Drawing for the job (mm, zero at the part's lowest x, y, z). A direction names the side the tool comes from. Coordinates: 2 decimals unless noted, no trailing zeros. Loops run counter-clockwise (first coordinate to the right, second up) from the corner with the lowest first, then second, coordinate; pieces in that order, holes last. Notation, with made-up numbers: (-39.75, -30.75) - (-5.75, -30.75) arc R13 cw to (-5.75, -6.75) - close; hole circle Ø1 at (28, -9.5). An arc over 180 degrees is marked (long way). Put each result on its own line as item: value.
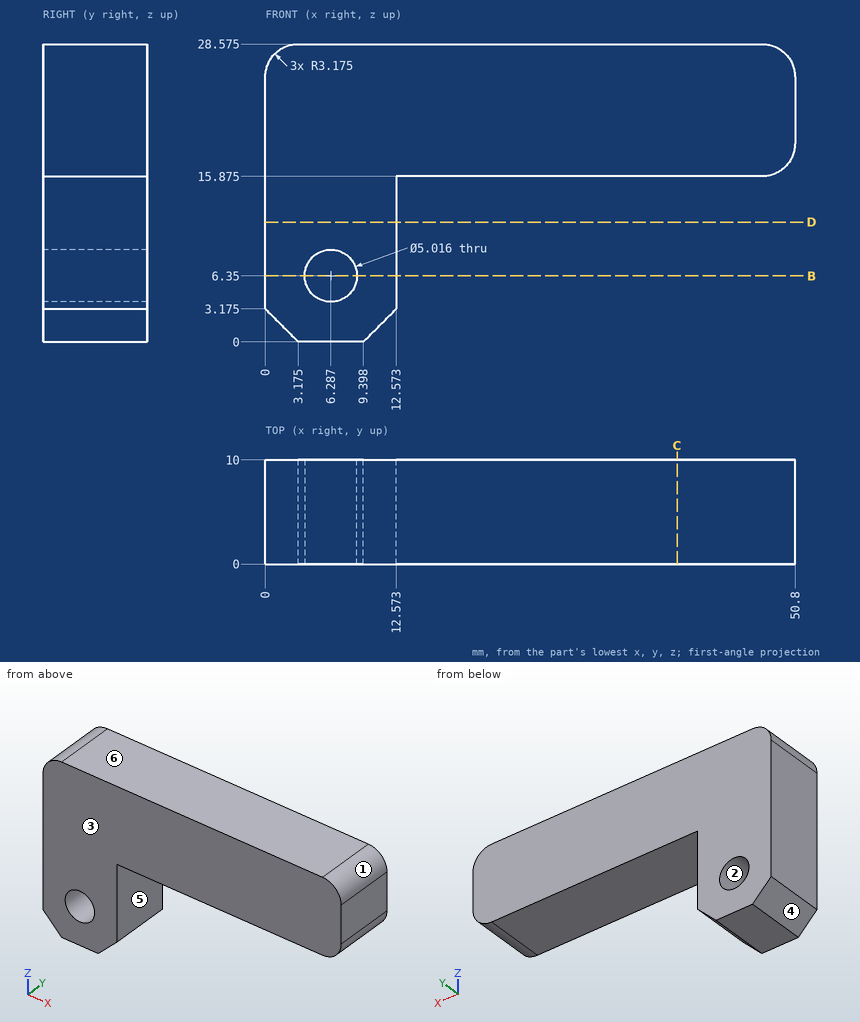
Q1. Slice it at D-D, the plane z = 11.5. Give the cut face in (x, y).
Determined:
outline: (0, 0) - (12.57, 0) - (12.57, 10) - (0, 10) - close
Q2. Tool access for the marked faces 5 and 6: list every direction of +Z, -Z, +X, -X, +Y, -Y with a clear straight run to the whole face (end or side of a thin tool).
Determined:
face 5: -Z, +X, +Y, -Y
face 6: +Z, +X, -X, +Y, -Y
Q3. Slice it at B-B, the plane z = 6.35. Give the cut face in (x, y) (1 decimal).
Determined:
outline: (0, 0) - (3.8, 0) - (3.8, 10) - (0, 10) - close; (8.8, 0) - (12.6, 0) - (12.6, 10) - (8.8, 10) - close
Q4. Slice it at C-C, the plane x = 39.5. Give the cut face in (y, z) (1 decimal), then the cut area to 3 significant figures.
Determined:
outline: (0, 15.9) - (10, 15.9) - (10, 28.6) - (0, 28.6) - close
area: 127 mm2
Q5. Mould opens along X. For the marked faces 1, 2, 3 and 4 say: +X half, -X half, draft (parallel to the pull), parting line (faces both ways), or undercut.
Determined:
face 1: +X half
face 2: undercut
face 3: draft
face 4: -X half
Q6. Wall check: L1, parallel to X at y = 8.25, z = 6.35 (1 decimal); L2, parallel to Z at x = 27.5, y = 8.5 (1 decimal); L3, parallel to Z at x = 4, y = 4.5 (1 decimal). Give the ranges that are in metal, low to high. Write a range as from..to.
Determined:
L1: 0..3.8, 8.8..12.6
L2: 15.9..28.6
L3: 0..5.3, 7.4..28.6
Q7. Pin check, flat tips, straight feed: pin 1 Ø1 at (y, z) = (4, 13) entering from +X; pin 2 Ø3 at (x, y) = (28.5, 6) entering from -Z (1 decimal); pin 3 Ø3 at (x, y) = (13, 6) entering from -Z. Stop position of each tip, or through.
Determined:
pin 1: x = 12.57
pin 2: z = 15.9
pin 3: z = 2.1
